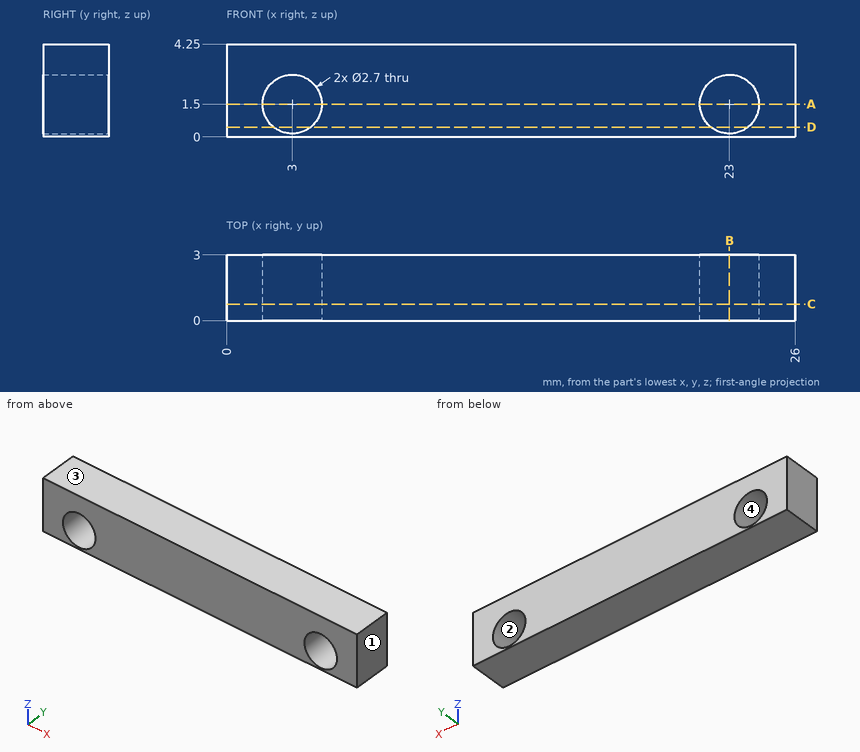
Here's the drawing with two shaded views (mm, measured from the low corner). I have some questions. Round coordinates to 2 decimals unless told otherwise and drop trailing zeros. Loops run counter-clockwise (first coordinate to the right, second up) from the corner with the lowest first, then second, coordinate; pieces in that order, holes last.
Item 1: If we mould it in two halves opening along X, with no side actions, what happens to the marked faces 1, 2, 3 and 4? For each: +X half, -X half, draft (parallel to the pull), parting line (faces both ways), or undercut.
Item 2: Will this pin go through, and if not, where does the flat tip stop? pin 1 Ø1.5 at (x, z) = (12.5, 2.5) entering from -Y.
Item 3: Suppose I cut it at D-D, the plane z = 0.45. Write out the boundary of the cut face in (x, y), then the cut area to 3 significant figures.
Item 4: Suppose I cut it at A-A, the plane z = 1.5. Write out the boundary of the cut face in (x, y).
Item 5: Suppose I cut it at C-C, the plane y = 0.75. Write out the boundary of the cut face in (x, z).
Item 6: Please list where these lines run through material, in increasing order: L1, parallel to X at y = 2.3, z = 1.45; L2, parallel to Z at x = 23, y = 2.2; L3, parallel to X at y = 2.8, z = 2.5.
Item 7: Suppose I cut it at B-B, the plane x = 23. Write out the boundary of the cut face in (y, z).
Reported:
1. face 1: +X half
1. face 2: undercut
1. face 3: draft
1. face 4: undercut
2. pin 1: stops at y = 0
3. outline: (0, 0) - (2.15, 0) - (2.15, 3) - (0, 3) - close; (3.85, 0) - (22.15, 0) - (22.15, 3) - (3.85, 3) - close; (23.85, 0) - (26, 0) - (26, 3) - (23.85, 3) - close
3. area: 67.8 mm2
4. outline: (0, 0) - (1.65, 0) - (1.65, 3) - (0, 3) - close; (4.35, 0) - (21.65, 0) - (21.65, 3) - (4.35, 3) - close; (24.35, 0) - (26, 0) - (26, 3) - (24.35, 3) - close
5. outline: (0, 0) - (26, 0) - (26, 4.25) - (0, 4.25) - close; hole circle Ø2.7 at (3, 1.5); hole circle Ø2.7 at (23, 1.5)
6. L1: x = 0 to 1.65, 4.35 to 21.65, 24.35 to 26
6. L2: z = 0 to 0.15, 2.85 to 4.25
6. L3: x = 0 to 2.09, 3.91 to 22.09, 23.91 to 26
7. outline: (0, 0) - (3, 0) - (3, 0.15) - (0, 0.15) - close; (0, 2.85) - (3, 2.85) - (3, 4.25) - (0, 4.25) - close
